Check sheet for the modelled part. Datum: model origin and axes. Units: mm. A direction names the side the tool comes from. Give positions to 0.01 mm unless a question says otherwise; leave off trailing zeros. Write each loop counter-clockwise with the first axis right and the second up, starting at its lowest first coordinate (ties: lowest second). Pieces come first, ordered by that corner, then holes. Notation, with made-up numbers: M 11,-9.5 L 16,-9.5 A21 cw 16,8.5 Z; hole C 57,-11.75 d7. An arc over 180 degrees is marked long. Write item = value, one per line. Start each with the question number.
1) Set-up check for faces 1 (the face through (-8.3, 11.5, -4.2)), 2 (the face through (0, 8, -17)), 3 (the face through (0, 8, 17)): record each of +Z, -Z, +X, -X, +Y, -Y from which the full face is reachable in a straight line by a thin tool's end or side.
2) Draft check along X on faces 4 (the face through (2.92, 2.71, -29.5)), 5 (the face through (0, 1.5, -6)), 6 (the face through (1.05, 2.71, -19.16)), 7 (the face through (-5.2, 0, 13.2)). Enter one of: pulls with the +X half, pulls with the -X half, needs draft (parallel to the pull), parting line crosses it, or undercut.
3) Sectioned sample at B-B, the plane y = 2.75. Record the cut outline in (x, z), then the cut area to 3 significant figures.
4) Sectioned sample at C-C, the plane x = 0. Record the cut outline in (y, z), then the cut area to 3 significant figures.
5) Scan lines: L1, parallel to Y at x = -14, z = 10.5; L2, parallel to Z at x = -2, y = 2; L3, parallel to X at y = 13.5, z = 1. Record each from-to range of solid material in increasing order.
6) Sectioned sample at D-D, the plane y = 10.75. Record the cut outline in (x, z).
7) Gauge pin test, flat ends, axial feed: pin 1 (6 mm diameter, centred on x = 10.5, z = -7, fed in from -Y); pin 2 (6.5 mm diameter, centred on x = 0, z = 22.5, fed in from -Y); pin 3 (1.5 mm diameter, centred on x = -14, y = 2, fed in from +Z); pin 4 (4.5 mm diameter, centred on x = 2.5, z = 20.5, fed in from +Y). Record the tip position at first contact, or that the pin passes through.
8) Sectioned sample at A-A, the plane z = 0. Record the cut outline in (x, y).
from build123d import *

# Parameters (mm, degrees)
SKETCH1_R      = 3.5
EXTRUDE1_DEPTH = 5.5
EXTRUDE2_DEPTH = 6
SKETCH3_R      = 9
EXTRUDE3_DEPTH = 4
SKETCH4_R      = 5
EXTRUDE4_DEPTH = 20
SKETCH5_R      = 14
EXTRUDE5_DEPTH = 1.5


with BuildPart() as part:
    # Sketch1 → Extrude1 (new body)
    with BuildSketch(Plane(origin=(0, 0, 0), x_dir=(1, 0, 0), z_dir=(0, 1, 0))):
        with BuildLine():
            Line((-9.142025191, 15.505591746), (-4.043990115, 28.123809223))
            ThreePointArc((-4.043990115, 28.123809223), (-2.940017716, 29.487109534), (-1.262434286, 30))
            Line((-1.262434286, 30), (1.262434286, 30))
            ThreePointArc((1.262434286, 30), (2.940017716, 29.487109534), (4.043990115, 28.123809223))
            Line((4.043990115, 28.123809223), (9.142025191, 15.505591746))
            ThreePointArc((9.142025191, 15.505591746), (18, 0), (9.142025191, -15.505591746))
            Line((9.142025191, -15.505591746), (4.043990115, -28.123809223))
            ThreePointArc((4.043990115, -28.123809223), (2.940017716, -29.487109534), (1.262434286, -30))
            Line((1.262434286, -30), (-1.262434286, -30))
            ThreePointArc((-1.262434286, -30), (-2.940017716, -29.487109534), (-4.043990115, -28.123809223))
            Line((-4.043990115, -28.123809223), (-9.142025191, -15.505591746))
            ThreePointArc((-9.142025191, -15.505591746), (-18, 0), (-9.142025191, 15.505591746))
        make_face()
        with Locations(Location((0, 22.5, 0), (0, 0, 270))):
            Circle(SKETCH1_R, mode=Mode.SUBTRACT)
        with Locations(Location((0, -22.5, 0), (0, 0, 270))):
            Circle(SKETCH1_R, mode=Mode.SUBTRACT)
    extrude(amount=EXTRUDE1_DEPTH)

    # Sketch2 → Extrude2 (add)
    with BuildSketch(Plane(origin=(0, 5.5, 0), x_dir=(1, 0, 0), z_dir=(0, 1, 0))):
        with BuildLine():
            ThreePointArc((2.819683898, -17.777777778), (18, 0), (2.819683898, 17.777777778))
            ThreePointArc((2.819683898, 17.777777778), (0, 17), (-2.819683898, 17.777777778))
            ThreePointArc((-2.819683898, 17.777777778), (-18, 0), (-2.819683898, -17.777777778))
            ThreePointArc((-2.819683898, -17.777777778), (0, -17), (2.819683898, -17.777777778))
        make_face()
    extrude(amount=EXTRUDE2_DEPTH)

    # Sketch3 → Extrude3 (add)
    with BuildSketch(Plane(origin=(0, 11.5, 0), x_dir=(1, 0, 0), z_dir=(0, 1, 0))):
        with Locations(Location((0, 0, 0), (0, 0, 270))):
            Circle(SKETCH3_R)
    extrude(amount=EXTRUDE3_DEPTH)

    # Sketch4 → Extrude4 (cut)
    with BuildSketch(Plane(origin=(0, 15.5, 0), x_dir=(1, 0, 0), z_dir=(0, 1, 0))):
        with Locations(Location((0, 0, 0), (0, 0, 270))):
            Circle(SKETCH4_R)
    extrude(amount=-EXTRUDE4_DEPTH, mode=Mode.SUBTRACT)

    # Sketch5 → Extrude5 (cut)
    with BuildSketch(Plane.XZ):
        with Locations(Location((0, 0, 0), (0, 0, 270))):
            Circle(SKETCH5_R)
    extrude(amount=-EXTRUDE5_DEPTH, mode=Mode.SUBTRACT)


solid = part.part
Data:
q1.face_1 = +Y
q1.face_2 = -Z, +Y
q1.face_3 = +Z, +Y
q2.face_4 = pulls with the +X half
q2.face_5 = undercut
q2.face_6 = undercut
q2.face_7 = needs draft
q3.outline = M -9.14,-15.51 L -4.04,-28.12 A3 ccw -1.26,-30 L 1.26,-30 A3 ccw 4.04,-28.12 L 9.14,-15.51 A18 ccw 9.14,15.51 L 4.04,28.12 A3 ccw 1.26,30 L -1.26,30 A3 ccw -4.04,28.12 L -9.14,15.51 A18 ccw Z; hole C 0,0 d10; hole C 0,-22.5 d7; hole C 0,22.5 d7
q3.area = 1,160 mm2
q4.outline = M 0,-30 L 5.5,-30 L 5.5,-26 L 0,-26 Z; M 0,-19 L 5.5,-19 L 5.5,-17 L 11.5,-17 L 11.5,-9 L 15.5,-9 L 15.5,-5 L 1.5,-5 L 1.5,-14 L 0,-14 Z; M 0,14 L 1.5,14 L 1.5,5 L 15.5,5 L 15.5,9 L 11.5,9 L 11.5,17 L 5.5,17 L 5.5,19 L 0,19 Z; M 0,26 L 5.5,26 L 5.5,30 L 0,30 Z
q4.area = 347 mm2
q5.L1 = 0 to 11.5
q5.L2 = -29.91 to -25.37, -19.63 to -4.58, 4.58 to 19.63, 25.37 to 29.91
q5.L3 = -8.94 to -4.9, 4.9 to 8.94
q6.outline = M -2.82,-17.78 A5.5 cw 2.82,-17.78 A18 ccw 2.82,17.78 A5.5 cw -2.82,17.78 A18 ccw Z; hole C 0,0 d10
q7.pin_1 = 0
q7.pin_2 = through
q7.pin_3 = 12.18
q7.pin_4 = 5.5
q8.outline = M -18,0 L -14,0 L -14,1.5 L -5,1.5 L -5,15.5 L -9,15.5 L -9,11.5 L -18,11.5 Z; M 5,1.5 L 14,1.5 L 14,0 L 18,0 L 18,11.5 L 9,11.5 L 9,15.5 L 5,15.5 Z
